```python
from build123d import *

# Parameters (mm, degrees)
LID_PLATE_START                        = 37.6
LID_PLATE_DEPTH                        = 2.4
TWO_SIDE_FASTENING_TABS_START          = 29
SKETCH_2_W                             = 8
SKETCH_2_H                             = 7.5
TWO_SIDE_FASTENING_TABS_DEPTH          = 8.6
M3_TAB_BORE_1_DEPTH                    = 3.8
M3_TAB_BORE_1_DEPTH_BACK               = 3.8
M3_TAB_BORE_1_START                    = -3.25
SKETCH_3_R                             = 1.6
M3_TAB_CAPTIVE_NUT_1_DEPTH             = 1.3
M3_TAB_CAPTIVE_NUT_1_DEPTH_BACK        = 1.3
M3_TAB_CAPTIVE_NUT_1_START             = -3.3
M3_TAB_NUT_LOADING_SLOT_1_DEPTH        = 1.3
M3_TAB_NUT_LOADING_SLOT_1_DEPTH_BACK   = 1.3
M3_TAB_NUT_LOADING_SLOT_1_START        = -3.3
SKETCH_5_W                             = 4.3
SKETCH_5_H                             = 6.7
M3_TAB_BORE_2_DEPTH                    = 3.8
M3_TAB_BORE_2_DEPTH_BACK               = 3.8
M3_TAB_BORE_2_START                    = 94.25
SKETCH_6_R                             = 1.6
M3_TAB_CAPTIVE_NUT_2_DEPTH             = 1.3
M3_TAB_CAPTIVE_NUT_2_DEPTH_BACK        = 1.3
M3_TAB_CAPTIVE_NUT_2_START             = 94.3
M3_TAB_NUT_LOADING_SLOT_2_DEPTH        = 1.3
M3_TAB_NUT_LOADING_SLOT_2_DEPTH_BACK   = 1.3
M3_TAB_NUT_LOADING_SLOT_2_START        = 94.3
SKETCH_8_W                             = 4.3
SKETCH_8_H                             = 6.7
SIDE_LOCATING_LIPS_START               = 35.6
SKETCH_9_W                             = 62
SKETCH_9_H                             = 1.2
SIDE_LOCATING_LIPS_DEPTH               = 2
LCD_VIEWING_WINDOW_DEPTH               = 144.896699059
LCD_VIEWING_WINDOW_DEPTH_BACK          = 144.896699059
LCD_MOUNTING_SPACERS_START             = 34.3
SKETCH_11_R                            = 2.1
LCD_MOUNTING_SPACERS_DEPTH             = 3.3
TWO_LCD_LOCATING_PINS_START            = 33.3
SKETCH_12_R                            = 0.8
TWO_LCD_LOCATING_PINS_DEPTH            = 1
TWO_BLIND_M1P6_LCD_PILOTS_DEPTH        = 1.45
TWO_BLIND_M1P6_LCD_PILOTS_DEPTH_BACK   = 1.45
TWO_BLIND_M1P6_LCD_PILOTS_START        = 35.75
SKETCH_13_R                            = 0.65
THREE_BUTTON_GUIDES_DEPTH              = 144.896699059
THREE_BUTTON_GUIDES_DEPTH_BACK         = 144.896699059
SKETCH_14_R                            = 2.95
BUTTON_RETAINER_BOSSES_START           = 35.6
SKETCH_15_R                            = 2.9
BUTTON_RETAINER_BOSSES_DEPTH           = 2
BUTTON_RETAINER_PILOT_HOLES_DEPTH      = 1.9
BUTTON_RETAINER_PILOT_HOLES_DEPTH_BACK = 1.9
BUTTON_RETAINER_PILOT_HOLES_START      = 37.5
SKETCH_16_R                            = 1.1
TOP_AIR_SLOTS_DEPTH                    = 144.896699059
TOP_AIR_SLOTS_DEPTH_BACK               = 144.896699059


with BuildPart() as part:
    # 草图1 → Lid_plate (new body)
    with BuildSketch(Plane.XY.offset(LID_PLATE_START)):
        with BuildLine():
            Line((-2.5, -9.5), (93.4, -9.5))
            ThreePointArc((93.4, -9.5), (94.460660172, -9.060660172), (94.9, -8))
            Line((94.9, -8), (94.9, 99))
            ThreePointArc((94.9, 99), (94.460660172, 100.060660172), (93.4, 100.5))
            Line((93.4, 100.5), (-2.5, 100.5))
            ThreePointArc((-2.5, 100.5), (-3.560660172, 100.060660172), (-4, 99))
            Line((-4, 99), (-4, -8))
            ThreePointArc((-4, -8), (-3.560660172, -9.060660172), (-2.5, -9.5))
        make_face()
    extrude(amount=LID_PLATE_DEPTH)

    # 草图2 → Two_side_fastening_tabs (add)
    with BuildSketch(Plane.XY.offset(TWO_SIDE_FASTENING_TABS_START)):
        with Locations((7, -3.25)):
            Rectangle(SKETCH_2_W, SKETCH_2_H)
        with Locations((84, 94.25)):
            Rectangle(SKETCH_2_W, SKETCH_2_H)
    extrude(amount=TWO_SIDE_FASTENING_TABS_DEPTH)

    # 草图3 → M3_tab_bore_1 (cut, two sides: drawn at the far end of the back side and taken through both)
    with BuildSketch(Plane(origin=(0, 0, 0), x_dir=(1, 0, 0), z_dir=(0, 1, 0)).offset(M3_TAB_BORE_1_START - M3_TAB_BORE_1_DEPTH_BACK)):
        with Locations(Location((7, -33.6, 0), (0, 0, 90))):
            Circle(SKETCH_3_R)
    extrude(amount=M3_TAB_BORE_1_DEPTH + M3_TAB_BORE_1_DEPTH_BACK, mode=Mode.SUBTRACT)

    # 草图4 → M3_tab_captive_nut_1 (cut, two sides: drawn at the far end of the back side and taken through both)
    with BuildSketch(Plane(origin=(0, 0, 0), x_dir=(1, 0, 0), z_dir=(0, 1, 0)).offset(M3_TAB_CAPTIVE_NUT_1_START - M3_TAB_CAPTIVE_NUT_1_DEPTH_BACK)):
        Polygon((9.875, -35.259882024), (7, -36.919764048), (4.125, -35.259882024), (4.125, -31.940117976), (7, -30.280235952), (9.875, -31.940117976), align=None)
    extrude(amount=M3_TAB_CAPTIVE_NUT_1_DEPTH + M3_TAB_CAPTIVE_NUT_1_DEPTH_BACK, mode=Mode.SUBTRACT)

    # 草图5 → M3_tab_nut_loading_slot_1 (cut, two sides: drawn at the far end of the back side and taken through both)
    with BuildSketch(Plane(origin=(0, 0, 0), x_dir=(1, 0, 0), z_dir=(0, 1, 0)).offset(M3_TAB_NUT_LOADING_SLOT_1_START - M3_TAB_NUT_LOADING_SLOT_1_DEPTH_BACK)):
        with Locations((9.15, -33.6)):
            Rectangle(SKETCH_5_W, SKETCH_5_H)
    extrude(amount=M3_TAB_NUT_LOADING_SLOT_1_DEPTH + M3_TAB_NUT_LOADING_SLOT_1_DEPTH_BACK, mode=Mode.SUBTRACT)

    # 草图6 → M3_tab_bore_2 (cut, two sides: drawn at the far end of the back side and taken through both)
    with BuildSketch(Plane(origin=(0, 0, 0), x_dir=(1, 0, 0), z_dir=(0, 1, 0)).offset(M3_TAB_BORE_2_START - M3_TAB_BORE_2_DEPTH_BACK)):
        with Locations(Location((84, -33.6, 0), (0, 0, 90))):
            Circle(SKETCH_6_R)
    extrude(amount=M3_TAB_BORE_2_DEPTH + M3_TAB_BORE_2_DEPTH_BACK, mode=Mode.SUBTRACT)

    # 草图7 → M3_tab_captive_nut_2 (cut, two sides: drawn at the far end of the back side and taken through both)
    with BuildSketch(Plane(origin=(0, 0, 0), x_dir=(1, 0, 0), z_dir=(0, 1, 0)).offset(M3_TAB_CAPTIVE_NUT_2_START - M3_TAB_CAPTIVE_NUT_2_DEPTH_BACK)):
        Polygon((86.875, -35.259882024), (84, -36.919764048), (81.125, -35.259882024), (81.125, -31.940117976), (84, -30.280235952), (86.875, -31.940117976), align=None)
    extrude(amount=M3_TAB_CAPTIVE_NUT_2_DEPTH + M3_TAB_CAPTIVE_NUT_2_DEPTH_BACK, mode=Mode.SUBTRACT)

    # 草图8 → M3_tab_nut_loading_slot_2 (cut, two sides: drawn at the far end of the back side and taken through both)
    with BuildSketch(Plane(origin=(0, 0, 0), x_dir=(1, 0, 0), z_dir=(0, 1, 0)).offset(M3_TAB_NUT_LOADING_SLOT_2_START - M3_TAB_NUT_LOADING_SLOT_2_DEPTH_BACK)):
        with Locations((81.85, -33.6)):
            Rectangle(SKETCH_8_W, SKETCH_8_H)
    extrude(amount=M3_TAB_NUT_LOADING_SLOT_2_DEPTH + M3_TAB_NUT_LOADING_SLOT_2_DEPTH_BACK, mode=Mode.SUBTRACT)

    # 草图9 → Side_locating_lips (add)
    with BuildSketch(Plane.XY.offset(SIDE_LOCATING_LIPS_START)):
        with Locations((46, -6.2)):
            Rectangle(SKETCH_9_W, SKETCH_9_H)
        with Locations((46, 97.2)):
            Rectangle(SKETCH_9_W, SKETCH_9_H)
    extrude(amount=SIDE_LOCATING_LIPS_DEPTH)

    # 草图10 → LCD_viewing_window (cut, two sides: drawn at the far end of the back side and taken through both)
    with BuildSketch(Plane.XY.offset(-LCD_VIEWING_WINDOW_DEPTH_BACK)):
        with BuildLine():
            Line((43.44, 6), (79.44, 6))
            ThreePointArc((79.44, 6), (79.793553391, 6.146446609), (79.94, 6.5))
            Line((79.94, 6.5), (79.94, 35.5))
            ThreePointArc((79.94, 35.5), (79.793553391, 35.853553391), (79.44, 36))
            Line((79.44, 36), (43.44, 36))
            ThreePointArc((43.44, 36), (43.086446609, 35.853553391), (42.94, 35.5))
            Line((42.94, 35.5), (42.94, 6.5))
            ThreePointArc((42.94, 6.5), (43.086446609, 6.146446609), (43.44, 6))
        make_face()
    extrude(amount=LCD_VIEWING_WINDOW_DEPTH + LCD_VIEWING_WINDOW_DEPTH_BACK, mode=Mode.SUBTRACT)

    # 草图11 → LCD_mounting_spacers (add)
    with BuildSketch(Plane.XY.offset(LCD_MOUNTING_SPACERS_START)):
        with Locations(Location((38.5, 6, 0), (0, 0, 180))):
            Circle(SKETCH_11_R)
        with Locations(Location((38.5, 36, 0), (0, 0, 180))):
            Circle(SKETCH_11_R)
        with Locations(Location((89.5, 6, 0), (0, 0, 180))):
            Circle(SKETCH_11_R)
        with Locations(Location((89.5, 36, 0), (0, 0, 180))):
            Circle(SKETCH_11_R)
    extrude(amount=LCD_MOUNTING_SPACERS_DEPTH)

    # 草图12 → Two_LCD_locating_pins (add)
    with BuildSketch(Plane.XY.offset(TWO_LCD_LOCATING_PINS_START)):
        with Locations((38.5, 6)):
            Circle(SKETCH_12_R)
        with Locations((89.5, 36)):
            Circle(SKETCH_12_R)
    extrude(amount=TWO_LCD_LOCATING_PINS_DEPTH)

    # 草图13 → Two_blind_M1p6_LCD_pilots (cut, two sides: drawn at the far end of the back side and taken through both)
    with BuildSketch(Plane.XY.offset(TWO_BLIND_M1P6_LCD_PILOTS_START - TWO_BLIND_M1P6_LCD_PILOTS_DEPTH_BACK)):
        with Locations((38.5, 36)):
            Circle(SKETCH_13_R)
        with Locations((89.5, 6)):
            Circle(SKETCH_13_R)
    extrude(amount=TWO_BLIND_M1P6_LCD_PILOTS_DEPTH + TWO_BLIND_M1P6_LCD_PILOTS_DEPTH_BACK, mode=Mode.SUBTRACT)

    # 草图14 → Three_button_guides (cut, two sides: drawn at the far end of the back side and taken through both)
    with BuildSketch(Plane.XY.offset(-THREE_BUTTON_GUIDES_DEPTH_BACK)):
        with Locations(Location((59, 54.355, 0), (0, 0, 180))):
            Circle(SKETCH_14_R)
        with Locations(Location((71, 54.355, 0), (0, 0, 180))):
            Circle(SKETCH_14_R)
        with Locations(Location((83, 54.355, 0), (0, 0, 180))):
            Circle(SKETCH_14_R)
    extrude(amount=THREE_BUTTON_GUIDES_DEPTH + THREE_BUTTON_GUIDES_DEPTH_BACK, mode=Mode.SUBTRACT)

    # 草图15 → Button_retainer_bosses (add)
    with BuildSketch(Plane.XY.offset(BUTTON_RETAINER_BOSSES_START)):
        with Locations((54, 48.5)):
            Circle(SKETCH_15_R)
        with Locations((88, 60.2)):
            Circle(SKETCH_15_R)
    extrude(amount=BUTTON_RETAINER_BOSSES_DEPTH)

    # 草图16 → Button_retainer_pilot_holes (cut, two sides: drawn at the far end of the back side and taken through both)
    with BuildSketch(Plane.XY.offset(BUTTON_RETAINER_PILOT_HOLES_START - BUTTON_RETAINER_PILOT_HOLES_DEPTH_BACK)):
        with Locations(Location((54, 48.5, 0), (0, 0, 180))):
            Circle(SKETCH_16_R)
        with Locations(Location((88, 60.2, 0), (0, 0, 180))):
            Circle(SKETCH_16_R)
    extrude(amount=BUTTON_RETAINER_PILOT_HOLES_DEPTH + BUTTON_RETAINER_PILOT_HOLES_DEPTH_BACK, mode=Mode.SUBTRACT)

    # 草图17 → Top_air_slots (cut, two sides: drawn at the far end of the back side and taken through both)
    with BuildSketch(Plane.XY.offset(-TOP_AIR_SLOTS_DEPTH_BACK)):
        with BuildLine():
            Line((10.2, 66), (25.8, 66))
            ThreePointArc((25.8, 66), (26.648528137, 66.351471863), (27, 67.2))
            Line((27, 67.2), (27, 67.4))
            ThreePointArc((27, 67.4), (26.648528137, 68.248528137), (25.8, 68.6))
            Line((25.8, 68.6), (10.2, 68.6))
            ThreePointArc((10.2, 68.6), (9.351471863, 68.248528137), (9, 67.4))
            Line((9, 67.4), (9, 67.2))
            ThreePointArc((9, 67.2), (9.351471863, 66.351471863), (10.2, 66))
        make_face()
        with BuildLine():
            Line((10.2, 71), (25.8, 71))
            ThreePointArc((25.8, 71), (26.648528137, 71.351471863), (27, 72.2))
            Line((27, 72.2), (27, 72.4))
            ThreePointArc((27, 72.4), (26.648528137, 73.248528137), (25.8, 73.6))
            Line((25.8, 73.6), (10.2, 73.6))
            ThreePointArc((10.2, 73.6), (9.351471863, 73.248528137), (9, 72.4))
            Line((9, 72.4), (9, 72.2))
            ThreePointArc((9, 72.2), (9.351471863, 71.351471863), (10.2, 71))
        make_face()
        with BuildLine():
            Line((10.2, 76), (25.8, 76))
            ThreePointArc((25.8, 76), (26.648528137, 76.351471863), (27, 77.2))
            Line((27, 77.2), (27, 77.4))
            ThreePointArc((27, 77.4), (26.648528137, 78.248528137), (25.8, 78.6))
            Line((25.8, 78.6), (10.2, 78.6))
            ThreePointArc((10.2, 78.6), (9.351471863, 78.248528137), (9, 77.4))
            Line((9, 77.4), (9, 77.2))
            ThreePointArc((9, 77.2), (9.351471863, 76.351471863), (10.2, 76))
        make_face()
        with BuildLine():
            Line((10.2, 81), (25.8, 81))
            ThreePointArc((25.8, 81), (26.648528137, 81.351471863), (27, 82.2))
            Line((27, 82.2), (27, 82.4))
            ThreePointArc((27, 82.4), (26.648528137, 83.248528137), (25.8, 83.6))
            Line((25.8, 83.6), (10.2, 83.6))
            ThreePointArc((10.2, 83.6), (9.351471863, 83.248528137), (9, 82.4))
            Line((9, 82.4), (9, 82.2))
            ThreePointArc((9, 82.2), (9.351471863, 81.351471863), (10.2, 81))
        make_face()
    extrude(amount=TOP_AIR_SLOTS_DEPTH + TOP_AIR_SLOTS_DEPTH_BACK, mode=Mode.SUBTRACT)


solid = part.part
```
The listing builds one solid part. Answer for the finished solid, in the listing's coordinates (mm). A direction names the side the tool comes from. Coordinates: 2 decimals unless noted, no trailing zeros. Loops run counter-clockwise (first coordinate to the right, second up) from the corner with the lowest first, then second, coordinate; pieces in that order, holes last. Notation, with made-up numbers: (86, 84) -> (97, 84) arc R24 cw to (97, 111) -> close; hole circle Ø7 at (50, -37.75). An arc over 180 degrees is marked (long way). Return JSON: item names as keys, results as strings. Group by question number.
(1) Which of the six approach directions +Z, -Z, +X, -X, +Y, -Y give full straight-line access (tool end or side, diameter ignored) to faces 4 (the cylindrical face through (55.34, 45.93, 36.59)), 5 (the flat face through (88.6, 6, 34.3)), 6 (the flat face through (9, -3, 30.25)), 7 (the flat face through (82, 94, 36.95)), 8 (the flat face through (18, 81, 39))?
(2) Determine the mould class of faces 1 (the flat face through (84, 94, 29)), 2 (the flat face through (9, -4.6, 34)), 3 (the cylindrical face through (73.3, 56.2, 38.8)) for opening direction Z: released by +Z, released by -Z, zero draft, split by the parting line, or undercut.
(3) A cutting plane is placed at B-B on x = 18. Write down the section's boundary in (y, z).
(4) A cutting plane is placed at D-D on y = 89. Write down the section's boundary in (x, z).
(5) A cutting plane is placed at A-A on y = 27.5. Write down the section's boundary in (x, z).
(6) Given pin 1 Ø1.3 at (x, y) = (53.5, -6.5) entering from -Z; pin 2 Ø5 at (x, z) = (57, 33) entering from -Y; pin 3 Ø2 at (x, y) = (88, 60.2) entering from -Z; pin 4 Ø2 at (x, y) = (37, 32) entering from -Z, each flat-ended and moving along its own axis, determine where each tip first touches the part or whether it passes through.
(7) A cutting plane is placed at C-C on x = 71. Write down the section's boundary in (y, z) (3 decimals), and give its area (3 significant figures).
(8) Find the intervals of material crossed by probe 1 along Y at (x, z) = (21, 38); probe 2 along Y at (x, z) = (54, 37.45); probe 3 along Y at (x, z) = (59, 38.8) (3 decimals), in increasing order. Write a range as from..to.
The answers:
{
 "1": {"face 4": "-Z", "face 5": "-Z, +X, -Y", "face 6": "+X", "face 7": "-X", "face 8": "+Z, -Z"},
 "2": {"face 1": "released by -Z", "face 2": "undercut", "face 3": "zero draft"},
 "3": {"outline": "(-9.5, 37.6) -> (-6.8, 37.6) -> (-6.8, 35.6) -> (-5.6, 35.6) -> (-5.6, 37.6) -> (66, 37.6) -> (66, 40) -> (-9.5, 40) -> close; (68.6, 37.6) -> (71, 37.6) -> (71, 40) -> (68.6, 40) -> close; (73.6, 37.6) -> (76, 37.6) -> (76, 40) -> (73.6, 40) -> close; (78.6, 37.6) -> (81, 37.6) -> (81, 40) -> (78.6, 40) -> close; (83.6, 37.6) -> (96.6, 37.6) -> (96.6, 35.6) -> (97.8, 35.6) -> (97.8, 37.6) -> (100.5, 37.6) -> (100.5, 40) -> (83.6, 40) -> close"},
 "4": {"outline": "(-4, 37.6) -> (94.9, 37.6) -> (94.9, 40) -> (-4, 40) -> close"},
 "5": {"outline": "(-4, 37.6) -> (42.94, 37.6) -> (42.94, 40) -> (-4, 40) -> close; (79.94, 37.6) -> (94.9, 37.6) -> (94.9, 40) -> (79.94, 40) -> close"},
 "6": {"pin 1": "stops at z = 35.6", "pin 2": "passes through", "pin 3": "stops at z = 39.4", "pin 4": "stops at z = 37.6"},
 "7": {"outline": "(-9.5, 37.6) -> (-6.8, 37.6) -> (-6.8, 35.6) -> (-5.6, 35.6) -> (-5.6, 37.6) -> (6, 37.6) -> (6, 40) -> (-9.5, 40) -> close; (36, 37.6) -> (51.405, 37.6) -> (51.405, 40) -> (36, 40) -> close; (57.305, 37.6) -> (96.6, 37.6) -> (96.6, 35.6) -> (97.8, 35.6) -> (97.8, 37.6) -> (100.5, 37.6) -> (100.5, 40) -> (57.305, 40) -> close", "area": "183 mm^2"},
 "8": {"probe 1": "y = -9.5..66, 68.6..71, 73.6..76, 78.6..81, 83.6..100.5", "probe 2": "y = -6.8..-5.6, 45.6..47.4, 49.6..51.4, 96.6..97.8", "probe 3": "y = -9.5..6, 36..51.405, 57.305..100.5"}
}
